```python
from build123d import *

# Parameters (mm, degrees)
SKETCH_1_W             = 1915
SKETCH_1_H             = 80
EXTRUDE_1_DEPTH        = 80
SKETCH_3_W             = 68
SKETCH_3_H             = 68
CUT_EXTRUDE_2_DEPTH    = 1919.339125389
FILLET_1_R             = 10
SKETCH_7_R             = 11
CUT_EXTRUDE_5_DEPTH    = 1919.339125389
PATTERN_LINEAR_3_COUNT = 2
PATTERN_LINEAR_3_PITCH = 1845.383428992


with BuildPart() as part:
    # 草图1 → 拉伸1 (new body)
    with BuildSketch(Plane.XY):
        with Locations((957.5, 40)):
            Rectangle(SKETCH_1_W, SKETCH_1_H)
    extrude(amount=EXTRUDE_1_DEPTH)

    # 草图3 → 拉伸2 (cut, through all)
    with BuildSketch(Plane.ZY):
        with Locations((46, 46)):
            Rectangle(SKETCH_3_W, SKETCH_3_H)
    extrude(amount=-CUT_EXTRUDE_2_DEPTH, mode=Mode.SUBTRACT)

    # 圆角1
    fillet_1_edges = [part.edges().sort_by_distance(p)[0] for p in [
        (957.5, 80, 12),
        (957.5, 12, 80),
    ]]
    fillet(fillet_1_edges, radius=FILLET_1_R)

    # 草图7 → 拉伸5 (cut, through all)
    with BuildSketch(Plane.XZ):
        with Locations(Location((34.75, 40, 0), (0, 0, 270))):
            Circle(SKETCH_7_R)
    cut_extrude_5 = extrude(amount=-CUT_EXTRUDE_5_DEPTH, mode=Mode.SUBTRACT)

    # 阵列(线性)3: 拉伸5 ×2
    with Locations(*[(i * PATTERN_LINEAR_3_PITCH, 0, 0) for i in range(1, PATTERN_LINEAR_3_COUNT)]):
        add(cut_extrude_5, mode=Mode.SUBTRACT)


solid = part.part
```
For this review, take the finished solid that the model builds, in its own axes (mm). A direction names the side the tool comes from. Round coordinates to 2 decimals unless told otherwise and drop trailing zeros. Loops run counter-clockwise (first coordinate to the right, second up) from the corner with the lowest first, then second, coordinate; pieces in that order, holes last.
(1) We need section B-B (y = 57). Give the boundary of the cut face in (x, z).
Returned:
outline: (0, 0) - (1915, 0) - (1915, 12) - (0, 12) - close
(2) We need section A-A (x = 557). Give the boundary of the cut face in (y, z).
Returned:
outline: (0, 0) - (80, 0) - (80, 2) arc R10 ccw to (70, 12) - (12, 12) - (12, 70) arc R10 ccw to (2, 80) - (0, 80) - close
(3) Tool access review of faces 1 (the flat face through (944, 41, 0)), 2 (the flat face through (944, 12, 41)): name each direction out of +Z, -Z, +X, -X, +Y, -Y from which nothing blocks a thin tool from reaching the whole face with its end or side.
Returned:
face 1: -Z, +X, -X, +Y, -Y
face 2: +Z, +X, -X, +Y
(4) Wall thickness on line 1 along X through (y, z) = (6, 40); line 2 along Z through (x, y) = (913.5, 51.5): over which ranges is each line inside the solid? List them lowest first.
Returned:
line 1: x = 0 to 23.75, 45.75 to 1869.13, 1891.13 to 1915
line 2: z = 0 to 12
(5) Clearance check with flat-ended pins moving along their axes: P1, Ø8, axis at x = 1652, y = 65, coming from the +Z side; P2, Ø3, axis at x = 1469.5, z = 51, coming from the +Y side; P3, Ø20, axis at x = 1880.13, z = 40, coming from the +Y side; P4, Ø8, axis at x = 1452, z = 23.5, coming from the -Y side. State where each tip first meets the part, or that it passes through.
Returned:
P1: stops at z = 12
P2: stops at y = 12
P3: passes through
P4: stops at y = 0
